```python
from build123d import *

# Parameters (mm, degrees)
SKETCH_1_R          = 6
EXTRUDE_1_DEPTH     = 20
SKETCH_3_R          = 1.65
CUT_EXTRUDE_2_DEPTH = 22.725560982
CUT_EXTRUDE_1_DEPTH = 22.725560982


with BuildPart() as part:
    # ｽｹｯﾁ1 → ﾎﾞｽ - 押し出し1 (new body)
    with BuildSketch(Plane(origin=(0, 0, 0), x_dir=(0, 0, -1), z_dir=(1, 0, 0))):
        Circle(SKETCH_1_R)
    extrude(amount=EXTRUDE_1_DEPTH)

    # ｽｹｯﾁ3 → ｶｯﾄ - 押し出し2 (cut, through all)
    with BuildSketch(Plane(origin=(20, 0, 0), x_dir=(0, 0, -1), z_dir=(1, 0, 0))):
        Circle(SKETCH_3_R)
    extrude(amount=-CUT_EXTRUDE_2_DEPTH, mode=Mode.SUBTRACT)

    # ｽｹｯﾁ2 → ｶｯﾄ - 押し出し1 (cut, through all)
    with BuildSketch(Plane(origin=(20, 0, 0), x_dir=(0, 0, -1), z_dir=(1, 0, 0))):
        with BuildLine():
            Line((2.397915762, -5.5), (-2.397915762, -5.5))
            ThreePointArc((-2.397915762, -5.5), (0, -6), (2.397915762, -5.5))
        make_face()
    extrude(amount=-CUT_EXTRUDE_1_DEPTH, mode=Mode.SUBTRACT)


solid = part.part
```
Work out the finished part from the listing and answer in its coordinate system (mm). Give positions to 0.01 mm unless a question says otherwise; leave off trailing zeros. Loops run counter-clockwise (first coordinate to the right, second up) from the corner with the lowest first, then second, coordinate; pieces in that order, holes last. Notation, with made-up numbers: (25.5, 81) -> (52.5, 81) arc R13 ccw to (52.5, 101) -> close; hole circle Ø2 at (85, -9). An arc over 180 degrees is marked (long way). Write item = value, one per line. Start each with the question number.
(1) Find section A-A on z = 0. Give the vertices of the cut face in (x, y), and give its area (3 significant figures).
(2) Find section B-B on y = 0. Give the vertices of the cut face in (x, z).
(3) Find the intervals of material crossed by probe 1 along Y at (x, z) = (13.5, 0); probe 2 along Z at (x, y) = (4.75, 1); probe 3 along Z at (x, y) = (1.75, -1.5), in increasing order. Write a range as from..to.
(4) Find section D-D on z = -2.75. Give the vertices of the cut face in (x, y), and give its area (3 significant figures).
(5) The mould has two halves that part along Z. Classify faces 1 (the cylindrical face through (10.14, 1.115, 1.216)), 2 (the flat face through (10, -5.5, 0)), 3 (the cylindrical face through (10, 6, 0)): +Z half, -Z half, draft (parallel to the pull), parting line (faces both ways), or undercut.
(6) Find section C-C on x = 15. Give the vertices of the cut face in (y, z).
(7) Given pin 1 Ø4 at (x, z) = (8, 4.5) entering from +Y; pin 2 Ø2 at (y, z) = (0, 0) entering from -X; pin 3 Ø1.5 at (x, y) = (5, 2.5) entering from -Z, each flat-ended and moving along its own axis, determine where each tip first touches the part or whether it passes through.
From the geometry:
q1.outline = (0, -5.5) -> (20, -5.5) -> (20, -1.65) -> (0, -1.65) -> close; (0, 1.65) -> (20, 1.65) -> (20, 6) -> (0, 6) -> close
q1.area = 164 mm^2
q2.outline = (0, -6) -> (20, -6) -> (20, -1.65) -> (0, -1.65) -> close; (0, 1.65) -> (20, 1.65) -> (20, 6) -> (0, 6) -> close
q3.probe_1 = -5.5..-1.65, 1.65..6
q3.probe_2 = -5.92..-1.31, 1.31..5.92
q3.probe_3 = -5.81..-0.69, 0.69..5.81
q4.outline = (0, -5.33) -> (20, -5.33) -> (20, 5.33) -> (0, 5.33) -> close
q4.area = 213 mm^2
q5.face_1 = undercut
q5.face_2 = draft
q5.face_3 = parting line
q6.outline = (-5.5, -2.4) arc R6 ccw (long way) to (-5.5, 2.4) -> close; hole circle Ø3.3 at (0, 0)
q7.pin_1 = 5.45
q7.pin_2 = through
q7.pin_3 = -5.74
